```python
from build123d import *

# Parameters (mm, degrees)
F0_R     = 1.5
F0_R_2   = 11
F0_R_3   = 2.5
F1_DEPTH = 40
F2_START = 30
F2_DEPTH = 10
F3_DEPTH = 10
F4_DEPTH = 2
F5_DEPTH = 22
F6_START = 5
F6_DEPTH = 30


with BuildPart() as f1:
    # F0 (on Front) → F1 (new body)
    with BuildSketch(Plane.XZ):
        Polygon((-14.3553390593, 21), (-21, 14.3553390593), (-21, -14.3553390593), (-14.3553390593, -21), (14.3553390593, -21), (21, -14.3553390593), (21, 14.3553390593), (14.3553390593, 21), align=None)
        with Locations((-15.5, -15.5)):
            Circle(F0_R, mode=Mode.SUBTRACT)
        with Locations((15.5, -15.5)):
            Circle(F0_R, mode=Mode.SUBTRACT)
        with Locations((-15.5, 15.5)):
            Circle(F0_R, mode=Mode.SUBTRACT)
        Circle(F0_R_2, mode=Mode.SUBTRACT)
        with Locations((15.5, 15.5)):
            Circle(F0_R, mode=Mode.SUBTRACT)
        Circle(F0_R_2)
        Circle(F0_R_3, mode=Mode.SUBTRACT)
        Circle(F0_R_3)
    extrude(amount=F1_DEPTH)

    # F0 (on Front) → F2 (join)
    with BuildSketch(Plane.XZ.offset(F2_START)):
        Polygon((-17.1837661841, 21), (-21, 17.1837661841), (-21, 14.3553390593), (-14.3553390593, 21), align=None)
        Polygon((-14.3553390593, -21), (-21, -14.3553390593), (-21, -17.1837661841), (-17.1837661841, -21), align=None)
        Polygon((21, -14.3553390593), (14.3553390593, -21), (17.1837661841, -21), (21, -17.1837661841), align=None)
        Polygon((17.1837661841, 21), (14.3553390593, 21), (21, 14.3553390593), (21, 17.1837661841), align=None)
    extrude(amount=F2_DEPTH)

    # F0 (on Front) → F3 (join)
    with BuildSketch(Plane.XZ):
        Polygon((17.1837661841, 21), (14.3553390593, 21), (21, 14.3553390593), (21, 17.1837661841), align=None)
        Polygon((-17.1837661841, 21), (-21, 17.1837661841), (-21, 14.3553390593), (-14.3553390593, 21), align=None)
        Polygon((-14.3553390593, -21), (-21, -14.3553390593), (-21, -17.1837661841), (-17.1837661841, -21), align=None)
        Polygon((21, -14.3553390593), (14.3553390593, -21), (17.1837661841, -21), (21, -17.1837661841), align=None)
    extrude(amount=F3_DEPTH)

    # F0 (on Front) → F4 (join)
    with BuildSketch(Plane.XZ):
        Circle(F0_R_2)
        Circle(F0_R_3, mode=Mode.SUBTRACT)
    extrude(amount=-F4_DEPTH)

    # F0 (on Front) → F5 (join)
    with BuildSketch(Plane.XZ):
        Circle(F0_R_3)
    extrude(amount=-F5_DEPTH)

    # F0 (on Front) → F6 (join)
    with BuildSketch(Plane.XZ.offset(F6_START)):
        with Locations((15.5, 15.5)):
            Circle(F0_R)
        with Locations((-15.5, 15.5)):
            Circle(F0_R)
        with Locations((-15.5, -15.5)):
            Circle(F0_R)
        with Locations((15.5, -15.5)):
            Circle(F0_R)
    extrude(amount=F6_DEPTH)


solid = f1.part
```
The model under review builds one solid part; all positions refer to its coordinate system, in mm. A direction names the side the tool comes from. Round coordinates to 2 decimals unless told otherwise and drop trailing zeros. Write each loop counter-clockwise with the first axis right and the second up, starting at its lowest first coordinate (ties: lowest second). Pieces come first, ordered by that corner, then holes. Notation, with made-up numbers: (-24, 59.25) -> (34, 59.25) arc R12 cw to (34, 71.25) -> close; hole circle Ø10 at (31.25, 10). An arc over 180 degrees is marked (long way). Use CSV: the item, a comma, the result in double quotes.
Q1. Consider section A-A (z = 0). Give the boundary of the cut face in (x, y), then the cut area to 3 significant figures.
Checks:
outline,"(-21, -40) -> (21, -40) -> (21, 0) -> (11, 0) -> (11, 2) -> (2.5, 2) -> (2.5, 22) -> (-2.5, 22) -> (-2.5, 2) -> (-11, 2) -> (-11, 0) -> (-21, 0) -> close"
area,"1,820 mm²"
Q2. Consider section B-B (y = -1). Give the boundary of the cut face in (x, z).
Checks:
outline,"(-21, -17.18) -> (-17.18, -21) -> (17.18, -21) -> (21, -17.18) -> (21, 17.18) -> (17.18, 21) -> (-17.18, 21) -> (-21, 17.18) -> close; hole circle Ø3 at (-15.5, -15.5); hole circle Ø3 at (-15.5, 15.5); hole circle Ø3 at (15.5, -15.5); hole circle Ø3 at (15.5, 15.5)"
Q3. Consider section C-C (y = -27). Give the boundary of the cut face in (x, z), then the cut area to 3 significant figures.
Checks:
outline,"(-21, -14.36) -> (-14.36, -21) -> (14.36, -21) -> (21, -14.36) -> (21, 14.36) -> (14.36, 21) -> (-14.36, 21) -> (-21, 14.36) -> close"
area,"1,680 mm²"
Q4. Mouldability with a two-part tool opening along Z and no side actions: class faces 4 (the flat face through (17.724, -19.86, 17.631)), 5 (the flat face through (-16, -5, 16)), 6 (the flat face through (0, 22, 0)) as released by +Z, released by -Z, zero draft, split by the parting line, or undercut.
Checks:
face 4,"released by +Z"
face 5,"undercut"
face 6,"zero draft"
Q5. For pin 1 Ø5 at (x, z) = (10, 4) entering from +Y; pin 2 Ø7.5 at (x, z) = (16.5, -19) entering from +Y; pin 3 Ø0.9 at (x, z) = (16, 16) entering from +Y, all flat-tipped, find the tip position at first contact; note any pin that passes through.
Checks:
pin 1,"y = 2"
pin 2,"y = 0"
pin 3,"y = -5"
Q6. For faces 1 (the cylindrical face through (14, -37.47, -15.43)), 2 (the flat face through (-17.631, -19.86, 17.724)), 3 (the cylindrical face through (-2.38, 0.99, -10.74)), list the 3-axis set-ups (+Z, -Z, +X, -X, +Y, -Y) from which the entire face can be reached by the end or side of a thin tool; tool diameter is ignored.
Checks:
face 1,"-Y"
face 2,"+Z, -X"
face 3,"+Y"
Q7. Consider section D-D (x = 15.5). Give the boundary of the cut face in (y, z), then the cut area to 3 significant figures.
Checks:
outline,"(-40, -21) -> (-30, -21) -> (-30, -19.86) -> (-10, -19.86) -> (-10, -21) -> (0, -21) -> (0, -17) -> (-5, -17) -> (-5, -14) -> (0, -14) -> (0, 14) -> (-5, 14) -> (-5, 17) -> (0, 17) -> (0, 21) -> (-10, 21) -> (-10, 19.86) -> (-30, 19.86) -> (-30, 21) -> (-40, 21) -> (-40, 17) -> (-35, 17) -> (-35, 14) -> (-40, 14) -> (-40, -14) -> (-35, -14) -> (-35, -17) -> (-40, -17) -> close"
area,"1,570 mm²"
Q8. To check wall thickness, follow probe 1 along Z at (x, y) = (15.5, -38.75); probe 2 along Y at (x, z) = (18, -18); probe 3 along Z at (x, y) = (-15, -38). State the ranges of each line that lie inside material, in increasing order. Write a range as [from, to].
Checks:
probe 1,"[-21, -17], [-14, 14], [17, 21]"
probe 2,"[-40, -30], [-10, 0]"
probe 3,"[-21, -16.91], [-14.09, 14.09], [16.91, 21]"
